Here's the drawing with two shaded views (mm, measured from the low corner). I have some questions. Give positions to 0.01 mm unless a question says otherwise; leave off trailing zeros. Loops run counter-clockwise (first coordinate to the right, second up) from the corner with the lowest first, then second, coordinate; pieces in that order, holes last. Notation, with made-up numbers: (65.25, 80) -> (107.25, 80) arc R20 cw to (107.25, 88) -> close; hole circle Ø2 at (29, 38). An arc over 180 degrees is marked (long way). Answer in a Markdown table with one row per item. Add a question column.
Item 1: For P1, Ø1, axis at x = 63.5, z = 57.5, coming from the -Y side, with a flat end and sliding along its axis, tell me the tip position at first contact or that it passes through.
Item 2: If we section it at B-B (y = 2.1): Give the number of separate pieces and of enclosed holes in the cut face, then the cut area to 3 significant figures.
Item 3: If I drill on line 1 (Z direction, x = 48, y = 1.65) (1 decimal); line 2 (Z direction, x = 49.5, y = 2.5) (1 decimal), over which ranges is the centre line in solid material (lowest first)?
Item 4: If we section it at A-A (x = 54): Write out the boundary of the cut face in (y, z) (1 decimal).
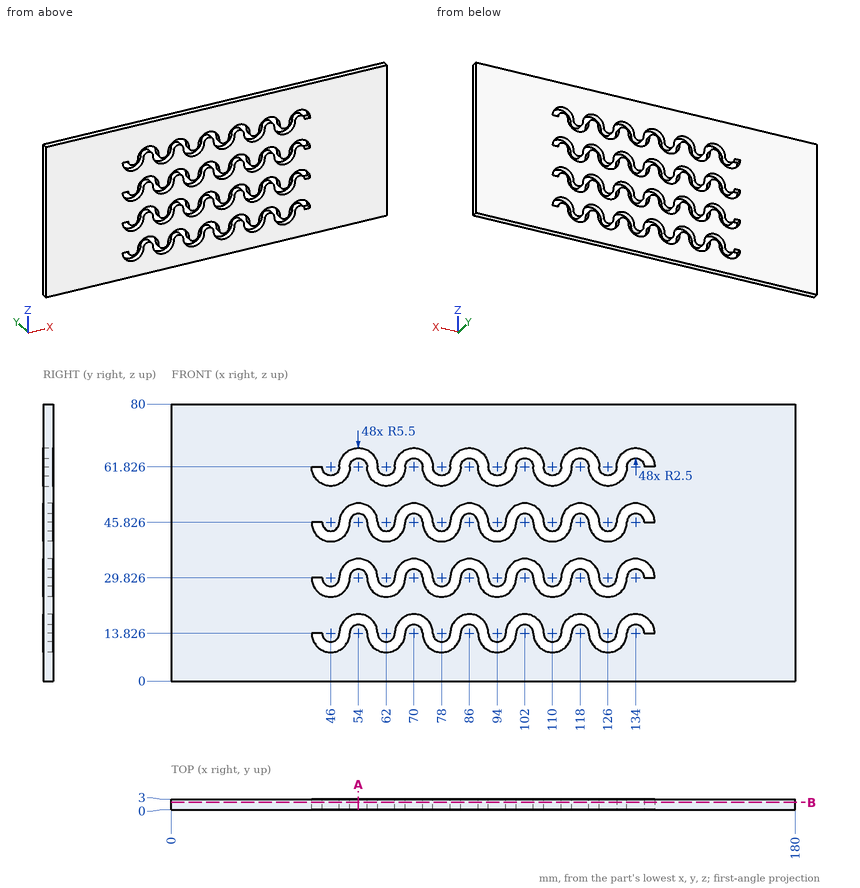
Recorded:
| question | item | result |
|---|---|---|
| 1 | P1 | passes through |
| 2 | separate pieces | 1 |
| 2 | enclosed holes | 4 |
| 2 | area | 12,600 mm^2 |
| 3 | line 1 | z = 0 to 8.7, 12.3 to 24.7, 28.3 to 40.7, 44.3 to 56.7, 60.3 to 80 |
| 3 | line 2 | z = 0 to 9.6, 17 to 25.6, 33 to 41.6, 49 to 57.6, 65 to 80 |
| 4 | outline | (0, 0) -> (3, 0) -> (3, 16.3) -> (0, 16.3) -> close; (0, 19.3) -> (3, 19.3) -> (3, 32.3) -> (0, 32.3) -> close; (0, 35.3) -> (3, 35.3) -> (3, 48.3) -> (0, 48.3) -> close; (0, 51.3) -> (3, 51.3) -> (3, 64.3) -> (0, 64.3) -> close; (0, 67.3) -> (3, 67.3) -> (3, 80) -> (0, 80) -> close |
